from build123d import *

# Parameters (mm, degrees)
SKETCH_1_W           = 20
SKETCH_1_H           = 20
SKETCH_1_W_2         = 11.5
SKETCH_1_H_2         = 11.5
EXTRUDE_1_DEPTH      = 7.5
EXTRUDE_2_DEPTH      = 20
SKETCH_4_W           = 6
SKETCH_4_H           = 17.5
CUT_EXTRUDE_1_DEPTH  = 33.882366095
SKETCH_5_R           = 2
CUT_EXTRUDE_2_DEPTH  = 35.820970693
SKETCH_6_OUTSIDE_W   = 31.014
SKETCH_6_OUTSIDE_H   = 48.514
SKETCH_6_OUTSIDE_W_2 = 18
SKETCH_6_OUTSIDE_H_2 = 37.5
CUT_EXTRUDE_5_DEPTH  = 33.882366095
EXTRUDE_3_DEPTH      = 15
CUT_EXTRUDE_6_DEPTH  = 75.578817368
CUT_EXTRUDE_9_DEPTH  = 37.120005833
SKETCH_12_W          = 2
SKETCH_12_H          = 2
CUT_EXTRUDE_10_DEPTH = 16
EXTRUDE_START        = -15
EXTRUDE_4_DEPTH      = 15
SKETCH_14_W          = 13
SKETCH_14_H          = 24
EXTRUDE_5_DEPTH      = 5
FILLET_3_R           = 5
CHAMFER_1_SIZE       = 0.5
CUT_EXTRUDE_11_DEPTH = 64
SKETCH_16_W          = 18
SKETCH_16_H          = 15
EXTRUDE_6_DEPTH      = 3
SKETCH_17_W          = 18
SKETCH_17_H          = 15
EXTRUDE_7_DEPTH      = 35
SKETCH_18_W          = 4.570911685
SKETCH_18_H          = 15.367720323
SKETCH_18_W_2        = 4.787102878
CUT_EXTRUDE_12_DEPTH = 66
SKETCH_19_R          = 2
CUT_EXTRUDE_13_DEPTH = 16


with BuildPart() as part:
    # 草图1 → 凸台-拉伸1 (new, symmetric)
    with BuildSketch(Plane(origin=(0, 0, 0), x_dir=(1, 0, 0), z_dir=(0, 1, 0))):
        Rectangle(SKETCH_1_W, SKETCH_1_H)
        Rectangle(SKETCH_1_W_2, SKETCH_1_H_2, mode=Mode.SUBTRACT)
    extrude(amount=EXTRUDE_1_DEPTH, both=True)

    # 草图3 → 凸台-拉伸2 (add)
    with BuildSketch(Plane.ZY.offset(10)):
        with BuildLine():
            Line((-10, -5), (-14.409830056, -5))
            ThreePointArc((-14.409830056, -5), (-27.5, 0), (-14.409830056, 5))
            Line((-14.409830056, 5), (-10, 5))
            Line((-10, 5), (-10, -5))
        make_face()
    extrude(amount=-EXTRUDE_2_DEPTH)

    # 草图4 → 切除-拉伸1 (cut, through all)
    with BuildSketch(Plane(origin=(0, 7.5, 0), x_dir=(1, 0, 0), z_dir=(0, 1, 0))):
        with Locations((-0.204363536, 18.75)):
            Rectangle(SKETCH_4_W, SKETCH_4_H)
    extrude(amount=-CUT_EXTRUDE_1_DEPTH, mode=Mode.SUBTRACT)

    # 草图5 → 切除-拉伸2 (cut, through all)
    with BuildSketch(Plane.ZY.offset(10)):
        with Locations((-20, 0)):
            Circle(SKETCH_5_R)
    extrude(amount=-CUT_EXTRUDE_2_DEPTH, mode=Mode.SUBTRACT)

    # 草图6 outside → 切除-拉伸5 (cut, through all)
    with BuildSketch(Plane(origin=(0, 7.5, 0), x_dir=(1, 0, 0), z_dir=(0, 1, 0))):
        with Locations((0, 8.75)):
            Rectangle(SKETCH_6_OUTSIDE_W, SKETCH_6_OUTSIDE_H)
        with Locations((0, 8.75)):
            Rectangle(SKETCH_6_OUTSIDE_W_2, SKETCH_6_OUTSIDE_H_2, mode=Mode.SUBTRACT)
    extrude(amount=-CUT_EXTRUDE_5_DEPTH, mode=Mode.SUBTRACT)


with BuildPart() as body_2:
    # 草图7 → 凸台-拉伸3 (new body)
    with BuildSketch(Plane.XZ.offset(7.5)):
        with BuildLine():
            Line((-9, 10), (-9, 22.751404539))
            ThreePointArc((-9, 22.751404539), (0, 69), (9, 22.751404539))
            Line((9, 22.751404539), (9, 10))
            Line((9, 10), (-9, 10))
        make_face()
    extrude(amount=-EXTRUDE_3_DEPTH)

    # 草图10 → 切除-拉伸6 (cut, through all)
    with BuildSketch(Plane(origin=(0, 7.5, 0), x_dir=(1, 0, 0), z_dir=(0, 1, 0))):
        with BuildLine():
            Line((-13.184152869, -27.388125792), (-20.784609691, -23))
            ThreePointArc((-20.784609691, -23), (0, -75.265491901), (20.784609691, -23))
            Line((20.784609691, -23), (14.677253023, -28.611643044))
            ThreePointArc((14.677253023, -28.611643044), (0.965186839, -23.021182599), (-13.184152869, -27.388125792))
        make_face()
    extrude(amount=-CUT_EXTRUDE_6_DEPTH, mode=Mode.SUBTRACT)


with BuildPart() as part_1:
    add(part.part)

    # Combine 1: union body 2
    add(body_2.part)

    # 草图11 → 切除-拉伸9 (cut, through all)
    with BuildSketch(Plane(origin=(0, 7.5, 0), x_dir=(1, 0, 0), z_dir=(0, 1, 0))):
        with BuildLine():
            Line((-7, -8.25), (7, -8.25))
            Line((7, -8.25), (7, -21))
            ThreePointArc((7, -21), (0, -20), (-7, -21))
            Line((-7, -21), (-7, -8.25))
        make_face()
    extrude(amount=-CUT_EXTRUDE_9_DEPTH, mode=Mode.SUBTRACT)

    # 草图12 → 切除-拉伸10 (cut)
    with BuildSketch(Plane(origin=(0, 7.5, 0), x_dir=(1, 0, 0), z_dir=(0, 1, 0))):
        with Locations((0, -23)):
            Rectangle(SKETCH_12_W, SKETCH_12_H)
    extrude(amount=-CUT_EXTRUDE_10_DEPTH, mode=Mode.SUBTRACT)

    # 草图13 → 凸台-拉伸4 (add)
    with BuildSketch(Plane.XZ.offset(7.5).offset(EXTRUDE_START)):
        with BuildLine():
            Line((-2, 20.080128411), (-2, 8.25))
            Line((-2, 8.25), (2, 8.25))
            Line((2, 8.25), (2, 20.080128411))
            ThreePointArc((2, 20.080128411), (0, 20), (-2, 20.080128411))
        make_face()
    extrude(amount=EXTRUDE_4_DEPTH)

    # 草图14 → 凸台-拉伸5 (add, symmetric)
    with BuildSketch(Plane(origin=(0, 0, 0), x_dir=(1, 0, 0), z_dir=(0, 1, 0))):
        with BuildLine():
            Line((-39.000369788, -25.608987518), (-10.391758029, -25.608987518))
            ThreePointArc((-10.391758029, -25.608987518), (-18.019377527, -32.37850906), (-21.774804011, -41.860269078))
            Line((-21.774804011, -41.860269078), (-22.000976364, -53.5))
            Line((-22.000976364, -53.5), (-39.000369788, -53.5))
            Line((-39.000369788, -53.5), (-39.000369788, -25.608987518))
        make_face()
        with Locations((-30.500369788, -39.5)):
            Rectangle(SKETCH_14_W, SKETCH_14_H, mode=Mode.SUBTRACT)
    extrude(amount=EXTRUDE_5_DEPTH, both=True)

    # 圆角3
    fillet_3_edges = [part_1.edges().sort_by_distance(p)[0] for p in [
        (-9, 0, 22.751404539),
        (9, 0, 22.751404539),
    ]]
    fillet(fillet_3_edges, radius=FILLET_3_R)

    # 倒角1
    # the kernel refuses this chamfer: 0.524377325, 0.5 mm, written as the material it takes off along each edge
    with BuildSketch(Plane(origin=(1, -8.868212894, 23.022739024), x_dir=(0.9983445219574435, 0, 0.05751708856995105), z_dir=(0, 1, 0))) as chamfer_1_piece_1:
        with BuildLine():
            Line((0.531447088, 0), (-CHAMFER_1_SIZE * 0.05751708857, CHAMFER_1_SIZE * 0.998344521957))
            Line((-CHAMFER_1_SIZE * 0.05751708857, CHAMFER_1_SIZE * 0.998344521957), (0, 0))
            ThreePointArc((0, 0), (0.273556674, 0.001603414), (0.531447088, 0))
        make_face()
    extrude(amount=17.736425787, mode=Mode.SUBTRACT)
    with BuildSketch(Plane(origin=(-1, -8.868212894, 23.022739024), x_dir=(-0.9983445219574435, 0, 0.05751708856995064), z_dir=(0, 1, 0))) as chamfer_1_piece_2:
        with BuildLine():
            Line((0.531447088, 0), (-CHAMFER_1_SIZE * 0.05751708857, -CHAMFER_1_SIZE * 0.998344521957))
            Line((-CHAMFER_1_SIZE * 0.05751708857, -CHAMFER_1_SIZE * 0.998344521957), (0, 0))
            ThreePointArc((0, 0), (0.273556674, -0.001603414), (0.531447088, 0))
        make_face()
    extrude(amount=17.736425787, mode=Mode.SUBTRACT)

    # 草图15 → 切除-拉伸11 (cut)
    with BuildSketch(Plane(origin=(0, 7.5, 0), x_dir=(1, 0, 0), z_dir=(0, 1, 0))):
        Polygon((-5.75, -5.75), (20.030525029, -5.75), (22.202632228, 33.927378984), (-42.503618679, 32.062961585), (-42.503618679, 30.637230633), (-36.910366482, 4.316043823), (-9, -5.75), align=None)
    extrude(amount=-CUT_EXTRUDE_11_DEPTH, mode=Mode.SUBTRACT)

    # 草图16 → 凸台-拉伸6 (add)
    with BuildSketch(Plane(origin=(0, 0, 5.75), x_dir=(-1, 0, 0), z_dir=(0, 0, -1))):
        Rectangle(SKETCH_16_W, SKETCH_16_H)
    extrude(amount=EXTRUDE_6_DEPTH)

    # 草图17 → 凸台-拉伸7 (add)
    with BuildSketch(Plane(origin=(0, 0, 2.75), x_dir=(-1, 0, 0), z_dir=(0, 0, -1))):
        Rectangle(SKETCH_17_W, SKETCH_17_H)
    extrude(amount=EXTRUDE_7_DEPTH)

    # 草图18 → 切除-拉伸12 (cut)
    with BuildSketch(Plane.XZ.offset(7.5)):
        with Locations((4.649601127, -4.742503957)):
            Rectangle(SKETCH_18_W, SKETCH_18_H)
        with Locations((-4.393551439, -4.742503957)):
            Rectangle(SKETCH_18_W_2, SKETCH_18_H)
    extrude(amount=-CUT_EXTRUDE_12_DEPTH, mode=Mode.SUBTRACT)

    # 草图19 → 切除-拉伸13 (cut)
    with BuildSketch(Plane(origin=(0, 0, -32.25), x_dir=(-1, 0, 0), z_dir=(0, 0, -1))):
        with Locations((-4, 4)):
            Circle(SKETCH_19_R)
        with Locations((4, 4)):
            Circle(SKETCH_19_R)
        with Locations(Location((4, -4, 0), (0, 0, 180))):
            Circle(SKETCH_19_R)
        with Locations(Location((-4, -4, 0), (0, 0, 180))):
            Circle(SKETCH_19_R)
    extrude(amount=-CUT_EXTRUDE_13_DEPTH, mode=Mode.SUBTRACT)


solid = part_1.part
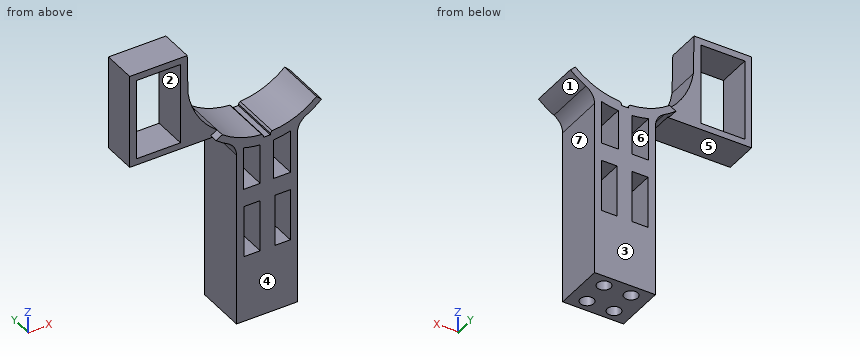
The listing builds one solid part. Answer for the finished solid, in the listing's coordinates (mm). Face numbers are marked on the shaded views. A direction names the side the tool comes from. Round coordinates to 2 decimals unless told otherwise and drop trailing zeros. Write each loop counter-clockwise with the first axis right and the second up, starting at its lowest first coordinate (ties: lowest second). Pieces come first, ordered by that corner, then holes. Notation, with made-up numbers: M 27.25,77.5 L 46.25,77.5 A12 ccw 46.25,89.5 Z; hole C 30.5,19.25 d9. An arc over 180 degrees is marked long. Write each question's results on one line, items separated by ' | '. Start each with the question number.
Item 1: For a pull along X with two mould halves and no side action, classify the marked faces 1, 2 and 3 as pulls with the +X half, pulls with the -X half, needs draft (parallel to the pull), parting line crosses it, or undercut.
Item 2: Straight lines are drawn through the part: L1, parallel to Y at x = 4, z = -28.25; L2, parallel to X at y = 4.75, z = 1; L3, parallel to Z at x = 5.5, y = -5. For each, find the intervals that lie inside material, in ascending order. Write a range as [from, to].
Item 3: Flat-ended cylindrical pins translate along their axes: pin 1 Ø6 at (y, z) = (0.5, 2.5) entering from -X; pin 2 Ø4.5 at (x, y) = (4, -4) entering from +Z; pin 3 Ø10 at (x, z) = (0, 31) entering from -Y; pin 4 Ø4 at (x, y) = (5, 0.5) entering from +Z. Find the tip coordinate at first contact, or state that the pin passes through.
Item 4: A cutting plane is placed at B-B on z = -21.5. Write down the section's boundary in (x, y).
Item 5: A cutting plane is placed at C-C on x = -3. Write down the section's boundary in (y, z).
Item 6: A cutting plane is placed at A-A on x = -31. Write down the section's boundary in (y, z).
Item 7: For the marked faces 4, 5, 6 and 7, determine the directions among +Z, -Z, +X, -X, +Y, -Y from which every point of the face is accessible in a straight line to the end or side of a thin tool.
Item 8: A cutting plane is placed at D-D on y = -4. State how many separate pieces and enclosed holes the cut face has, and give its area (3 significant figures).
Check sheet entries:
1) face 1: pulls with the +X half | face 2: undercut | face 3: needs draft
2) L1: [-7.5, -6], [-2, 2], [6, 7.5] | L2: [-9, -6.79], [-2, 2.36], [6.94, 9] | L3: [-16.25, -12.43], [2.94, 8.25], [20.61, 23.7]
3) pin 1: x = -9 | pin 2: z = 23.91 | pin 3: through | pin 4: z = 24.14
4) outline: M -9,-7.5 L 9,-7.5 L 9,7.5 L -9,7.5 Z; hole C -4,-4 d4; hole C -4,4 d4; hole C 4,-4 d4; hole C 4,4 d4
5) outline: M -7.5,-32.25 L -5.73,-32.25 L -5.73,-16.25 L -2.27,-16.25 L -2.27,-32.25 L 2.27,-32.25 L 2.27,-16.25 L 5.73,-16.25 L 5.73,-32.25 L 7.5,-32.25 L 7.5,-12.43 L -7.5,-12.43 Z; M -7.5,2.94 L 7.5,2.94 L 7.5,8.25 L -7.5,8.25 Z; M -7.5,20.18 L 7.5,20.18 L 7.5,23.21 L -7.5,23.21 Z
6) outline: M -5,25.61 L 5,25.61 L 5,27.5 L -5,27.5 Z; M -5,51.5 L 5,51.5 L 5,53.5 L -5,53.5 Z
7) face 4: +Z, -Z, +X, -X, -Y | face 5: -Z, -X, +Y, -Y | face 6: +Y, -Y | face 7: -Z, +X, +Y, -Y
8) separate pieces: 1 | enclosed holes: 5 | area: 864 mm²
